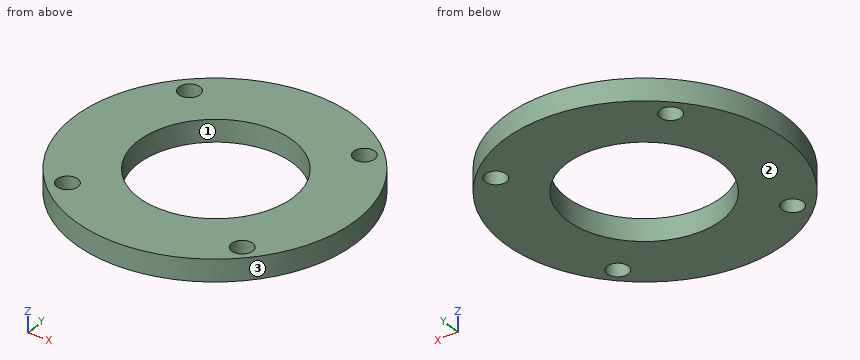
from build123d import *

# Parameters (mm, degrees)
SKETCH1_R          = 20.5
EXTRUDE1_DEPTH     = 3.2
SKETCH2_R          = 11.25
CUT_EXTRUDE1_DEPTH = 61.417603842
SKETCH3_R          = 1.55
CUT_EXTRUDE2_DEPTH = 61.417603842


with BuildPart() as part:
    # Sketch1 → Extrude1 (new body)
    with BuildSketch(Plane.XY):
        with Locations((22.085163637, 22.23816435)):
            Circle(SKETCH1_R)
    extrude(amount=EXTRUDE1_DEPTH)

    # Sketch2 → Cut-Extrude1 (cut, through all)
    with BuildSketch(Plane.XY.offset(3.2)):
        with Locations((22.225, 22.225)):
            Circle(SKETCH2_R)
    extrude(amount=-CUT_EXTRUDE1_DEPTH, mode=Mode.SUBTRACT)

    # Sketch3 → Cut-Extrude2 (cut, through all)
    with BuildSketch(Plane.XY.offset(3.2)):
        with Locations((34.925, 34.925)):
            Circle(SKETCH3_R)
        with Locations((9.525, 34.925)):
            Circle(SKETCH3_R)
        with Locations((34.925, 9.525)):
            Circle(SKETCH3_R)
        with Locations((9.525, 9.525)):
            Circle(SKETCH3_R)
    extrude(amount=-CUT_EXTRUDE2_DEPTH, mode=Mode.SUBTRACT)


solid = part.part
Source: CAD feature listing. Evaluate the final solid. Frame: model axes, mm. Face numbers are marked on the shaded views. Give positions to 0.01 mm unless a question says otherwise; leave off trailing zeros. Write each loop counter-clockwise with the first axis right and the second up, starting at its lowest first coordinate (ties: lowest second). Pieces come first, ordered by that corner, then holes. Notation, with made-up numbers: (-29, -34.5) -> (-10, -34.5) arc R21 ccw to (-10, 0.5) -> close; hole circle Ø11 at (-31.75, 41.25). An arc over 180 degrees is marked (long way). Return JSON: item names as keys, results as strings. Group by question number.
1. Section C-C, the plane y = 8.5. Output: boundary loops of the cut face in (x, z), then the cut area to 3 significant figures.
2. Section A-A, the plane y = 28.5. Output: boundary loops of the cut face in (x, z), then the cut area to 3 significant figures.
3. Material intervals for line 1 (X direction, y = 9, z = 1.5); line 2 (X direction, y = 34, z = 2.4); line 3 (X direction, y = 22, z = 0.35), sorted ascending. Write a range as from..to.
4. Pin query (flat end, axial travel): pin 1 Ø1 at (y, z) = (28, 2.5) entering from +X; pin 2 Ø1.5 at (y, z) = (11, 2) entering from +X. Return the tip coordinate at first contact, or that it passes through.
5. Section D-D, the plane z = 1. Output: boundary loops of the cut face in (x, y) (3 decimals), then the cut area to 3 significant figures.
6. Section B-B, the plane x = 27. Output: boundary loops of the cut face in (y, z), then the cut area to 3 significant figures.
7. Mould query, pull axis X, two halves, no side actions, for the marked faces 1, 2 and 3. Classes: +X half, -X half, draft (parallel to the pull), parting line (faces both ways), or undercut.
Determined:
{
 "1": {"outline": "(6.87, 0) -> (8.36, 0) -> (8.36, 3.2) -> (6.87, 3.2) -> close; (10.69, 0) -> (33.76, 0) -> (33.76, 3.2) -> (10.69, 3.2) -> close; (36.09, 0) -> (37.3, 0) -> (37.3, 3.2) -> (36.09, 3.2) -> close", "area": "82.5 mm2"},
 "2": {"outline": "(2.56, 0) -> (12.89, 0) -> (12.89, 3.2) -> (2.56, 3.2) -> close; (31.56, 0) -> (41.61, 0) -> (41.61, 3.2) -> (31.56, 3.2) -> close", "area": "65.2 mm2"},
 "3": {"line 1": "x = 6.43..8.07, 10.98..33.47, 36.38..37.74", "line 2": "x = 5.3..8.28, 10.77..33.68, 36.17..38.88", "line 3": "x = 1.59..10.98, 33.47..42.58"},
 "4": {"pin 1": "stops at x = 41.9", "pin 2": "stops at x = 39.7"},
 "5": {"outline": "circle Ø41 at (22.085, 22.238); hole circle Ø3.1 at (9.525, 9.525); hole circle Ø3.1 at (9.525, 34.925); hole circle Ø22.5 at (22.225, 22.225); hole circle Ø3.1 at (34.925, 9.525); hole circle Ø3.1 at (34.925, 34.925)", "area": "892 mm2"},
 "6": {"outline": "(2.34, 0) -> (12.04, 0) -> (12.04, 3.2) -> (2.34, 3.2) -> close; (32.41, 0) -> (42.14, 0) -> (42.14, 3.2) -> (32.41, 3.2) -> close", "area": "62.2 mm2"},
 "7": {"face 1": "undercut", "face 2": "draft", "face 3": "parting line"}
}
